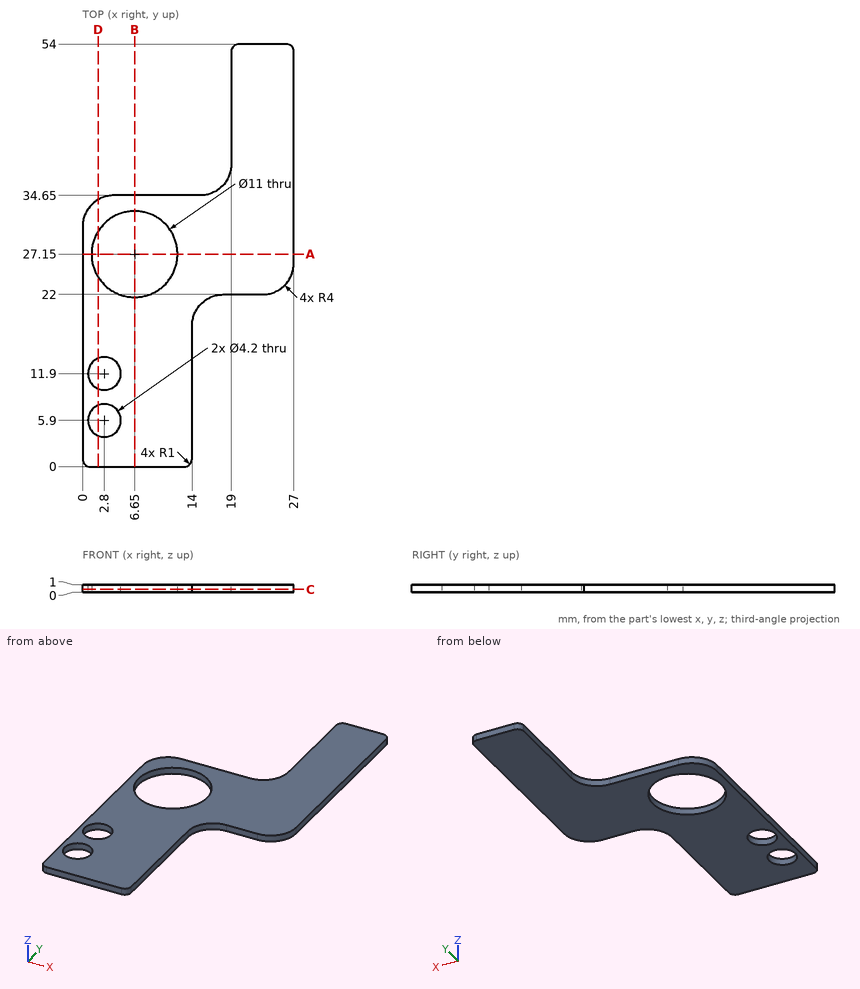
Geometry check sheet. Reference: drawing and pictorial views, mm from the part's lowest x, y, z. Give positions to 0.01 mm unless a question says otherwise; leave off trailing zeros. Order: outer loops, then holes, each group sorted by start corner. A loop starts at its lowest first (then second) coordinate and runs counter-clockwise, first axis right, second up. Notation, with made-up numbers: M 18,-29.75 L 67,-29.75 A21 ccw 67,-23.75 Z; hole C 36,64.25 d6. An arc over 180 degrees is marked long. Answer in a Markdown table with one row per item.
1) Cross-section at A-A, the plane y = 27.15. Enter the section's corners in (x, z).
Filled sheet:
| item | result |
|---|---|
| outline | M 0,0 L 1.15,0 L 1.15,1 L 0,1 Z; M 12.15,0 L 27,0 L 27,1 L 12.15,1 Z |
2) Cross-section at B-B, the plane x = 6.65. Enter the section's corners in (y, z).
Filled sheet:
| item | result |
|---|---|
| outline | M 0,0 L 21.65,0 L 21.65,1 L 0,1 Z; M 32.65,0 L 34.65,0 L 34.65,1 L 32.65,1 Z |
3) Cross-section at C-C, the plane z = 0.4. Enter the section's corners in (x, y), plus the area to 3 significant figures.
Filled sheet:
| item | result |
|---|---|
| outline | M 0,1 A1 ccw 1,0 L 13,0 A1 ccw 14,1 L 14,18 A4 cw 18,22 L 23,22 A4 ccw 27,26 L 27,53 A1 ccw 26,54 L 20,54 A1 ccw 19,53 L 19,38.65 A4 cw 15,34.65 L 4,34.65 A4 ccw 0,30.65 Z; hole C 2.8,5.9 d4.2; hole C 2.8,11.9 d4.2; hole C 6.65,27.15 d11 |
| area | 681 mm2 |
4) Gauge pin test, flat end, axial feed: P1, Ø0.5, axis at x = 20.5, z = 0.5, coming from the -Y side. Record the tip position at first contact, or that the pin passes through.
Filled sheet:
| item | result |
|---|---|
| P1 | stops at y = 22 |
5) Thickness scan on L1, parallel to Y at x = 2.75, z = 0.8; L2, parallel to Y at x = 6.65, z = 0.55; L3, parallel to Y at x = 2.8, z = 0.45. Record the ranges inside material, lowest first. Write a range as [from, to].
Filled sheet:
| item | result |
|---|---|
| L1 | y = [0, 3.8], [8, 9.8], [14, 23.27], [31.03, 34.45] |
| L2 | y = [0, 21.65], [32.65, 34.65] |
| L3 | y = [0, 3.8], [8, 9.8], [14, 23.22], [31.08, 34.47] |
6) Cross-section at D-D, the plane x = 2. Enter the section's corners in (y, z), plus the area to 3 significant figures.
Filled sheet:
| item | result |
|---|---|
| outline | M 0,0 L 3.96,0 L 3.96,1 L 0,1 Z; M 7.84,0 L 9.96,0 L 9.96,1 L 7.84,1 Z; M 13.84,0 L 24.21,0 L 24.21,1 L 13.84,1 Z; M 30.09,0 L 34.11,0 L 34.11,1 L 30.09,1 Z |
| area | 20.5 mm2 |
